```python
from build123d import *

# Parameters (mm, degrees)
F0_R     = 31.75
F1_DEPTH = 5.08
F2_R     = 1
F3_DEPTH = 5.081
F4_R     = 0.897754
F5_DEPTH = 5.081


with BuildPart() as f1:
    # F0 (on Top) → F1 (new body)
    with BuildSketch(Plane.XY):
        Circle(F0_R)
    extrude(amount=F1_DEPTH)

    # F2 (on face) → F3 (cut, through all)
    with BuildSketch(Plane(origin=(0, 0, 0), x_dir=(1, 0, 0), z_dir=(0, 0, -1))):
        Circle(F2_R)
    extrude(amount=-F3_DEPTH, mode=Mode.SUBTRACT)

    # F4 (on face) → F5 (cut, through all)
    with BuildSketch(Plane.XY.offset(5.08)):
        with Locations((2.140864, 7.005748)):
            Circle(F4_R)
    extrude(amount=-F5_DEPTH, mode=Mode.SUBTRACT)


solid = f1.part
```
For this review, take the finished solid that the model builds, in its own axes (mm). Round coordinates to 2 decimals unless told otherwise and drop trailing zeros. Write each loop counter-clockwise with the first axis right and the second up, starting at its lowest first coordinate (ties: lowest second). Pieces come first, ordered by that corner, then holes.
1) For line 1 along Y through (x, z) = (0, 1.35); line 2 along X through (y, z) = (2, 2.3); line 3 along Y through (x, z) = (8, 0.45), list the stretches that pass through material, from the lowest coordinate up.
Answer below:
line 1: y = -31.75 to -1, 1 to 31.75
line 2: x = -31.69 to 31.69
line 3: y = -30.73 to 30.73
2) Mouldability with a two-part tool opening along Y and no side actions: class faces 1 (the face through (-6.883, -30.995, 2.504)), 2 (the face through (7, 0, 0)), 3 (the face through (1.4, 6.5, 2.6)) as +Y half, -Y half, draft (parallel to the pull), parting line (faces both ways), or undercut.
Answer below:
face 1: parting line
face 2: draft
face 3: undercut
3) Take a section at C-C on z = 2.8. Give the boundary of the cut face in (x, y).
Answer below:
outline: circle Ø63.5 at (0, 0); hole circle Ø2 at (0, 0); hole circle Ø1.8 at (2.14, 7.01)
4) Insertion check: pin 1 Ø8 at (x, y) = (-15, -13.5) entering from -Z; pin 2 Ø1.5 at (x, z) = (13, 1) entering from -Y; pin 3 Ø2 at (x, z) = (1.5, 3.5) entering from -Y; pin 4 Ø1.5 at (y, z) = (-6.5, 4.5) entering from +X (3 decimals). Each pin has a flat end and moves straight along its axis. Give the tip position at first contact, or say it passes through.
Answer below:
pin 1: stops at z = 0
pin 2: stops at y = -29.29
pin 3: stops at y = -31.75
pin 4: stops at x = 31.225
5) Take a section at D-D on y = 21. Give the boundary of the cut face in (x, z), then the cut area to 3 significant figures.
Answer below:
outline: (-23.81, 0) - (23.81, 0) - (23.81, 5.08) - (-23.81, 5.08) - close
area: 242 mm2
6) Take a section at A-A on x = 0. Give the boundary of the cut face in (y, z), then the cut area to 3 significant figures.
Answer below:
outline: (-31.75, 0) - (-1, 0) - (-1, 5.08) - (-31.75, 5.08) - close; (1, 0) - (31.75, 0) - (31.75, 5.08) - (1, 5.08) - close
area: 312 mm2
